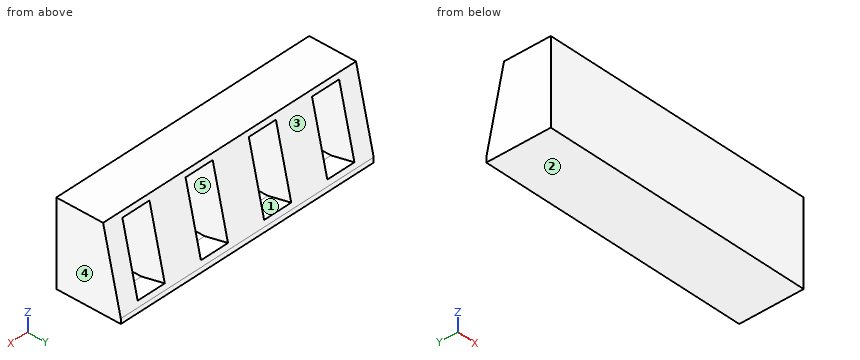
from build123d import *

# Parameters (mm, degrees)
SKETCH1_W           = 711.2
SKETCH1_H           = 167.132
BOSS_EXTRUDE2_DEPTH = 203.2
CUT_EXTRUDE3_DEPTH  = 919.48
SKETCH6_W           = 76.2
SKETCH6_H           = 180.34
CUT_EXTRUDE5_DEPTH  = 114.3
SKETCH7_W           = 711.2
SKETCH7_H           = 167.132
BOSS_EXTRUDE3_DEPTH = 12.7


with BuildPart() as part:
    # Sketch1 → Boss-Extrude2 (new body)
    with BuildSketch(Plane.XY):
        with Locations((355.6, 83.566)):
            Rectangle(SKETCH1_W, SKETCH1_H)
    extrude(amount=BOSS_EXTRUDE2_DEPTH)

    # Sketch5 → Cut-Extrude3 (cut)
    with BuildSketch(Plane(origin=(711.2, 0, 0), x_dir=(0, 0, -1), z_dir=(1, 0, 0))):
        Polygon((0, 167.132), (-203.2, 121.275720121), (-203.2, 167.132), align=None)
    extrude(amount=-CUT_EXTRUDE3_DEPTH, mode=Mode.SUBTRACT)

    # Sketch6 → Cut-Extrude5 (cut)
    with BuildSketch(Plane(origin=(0, 159.032892036, 35.88905909), x_dir=(1, 0, 0), z_dir=(0, 0.9754694514544971, 0.22013484340072725))):
        with Locations((266.7, -67.363402116)):
            Rectangle(SKETCH6_W, SKETCH6_H)
        with Locations((88.9, -67.363402116)):
            Rectangle(SKETCH6_W, SKETCH6_H)
        with Locations((444.5, -67.363402116)):
            Rectangle(SKETCH6_W, SKETCH6_H)
        with Locations((622.3, -67.363402116)):
            Rectangle(SKETCH6_W, SKETCH6_H)
    extrude(amount=-CUT_EXTRUDE5_DEPTH, mode=Mode.SUBTRACT)

    # Sketch7 → Boss-Extrude3 (add)
    with BuildSketch(Plane(origin=(0, 0, 0), x_dir=(-1, 0, 0), z_dir=(0, 0, -1))):
        with Locations((-355.6, 83.566)):
            Rectangle(SKETCH7_W, SKETCH7_H)
    extrude(amount=BOSS_EXTRUDE3_DEPTH)


solid = part.part
Could you check a few things on this model? Use its own coordinates, in mm. Face numbers are marked on the shaded views. A direction names the side the tool comes from. Coordinates: 2 decimals unless noted, no trailing zeros. Order: outer loops, then holes, each group sorted by start corner. A loop starts at its lowest first (then second) coordinate and runs counter-clockwise, first axis right, second up. Notation, with made-up numbers: (68.25, 85.25) - (92.25, 85.25) arc R13 ccw to (92.25, 100.25) - close; hole circle Ø11 at (11, -1.75). An arc over 180 degrees is marked (long way). Answer in a Markdown table with one row per item. Add a question column.
(1) I need wall thicknesses on L1, parallel to X at y = 81.5, z = 98.5; L2, parallel to Z at x = 298, y = 105; L3, parallel to Z at x = 103, y = 86. Which ranges of each line are inside material? Lowest first, please.
(2) If we section it at C-C, the plane z = 57.5: Please give me the cut outline in (x, y).
(3) If we section it at A-A, the plane x = 253: Please give me the cut outline in (y, z).
(4) If we section it at D-D, the plane y = 144: Please give me the cut outline in (x, z), then the cut area to 3 significant figures.
(5) If we mould it in two halves opening along X, with no side actions, what happens to the marked faces 3, 4 and 5? For each: released by +X, released by -X, zero draft, split by the parting line, or undercut.
(6) On a 3-axis mill with a long thin cutter (end or side, diameter ignored), from which of +Z, -Z, +X, -X, +Y, -Y can I reach the whole of each face in a straight line? I mean the marked faces 1 and 2. Say none if no direction works.
(7) If we section it at B-B, the plane y = 79.5: Please give me the cut outline in (x, z).
(8) Will these pins go through, and if not, where does the flat tip stop? pin 1 (10 mm diameter, centred on x = 301, z = 172, fed in from +Y); pin 2 (4 mm diameter, centred on x = 550.5, z = 10, fed in from +Y); pin 3 (12 mm diameter, centred on y = 141, z = 145.5, fed in from -X); pin 4 (1.5 mm diameter, centred on x = 520, z = 103, fed in from +Y).
Results are:
| question | item | result |
|---|---|---|
| 1 | L1 | x = 0 to 50.8, 127 to 228.6, 304.8 to 406.4, 482.6 to 584.2, 660.4 to 711.2 |
| 1 | L2 | z = -12.7 to 0.32, 185.19 to 203.2 |
| 1 | L3 | z = -12.7 to 0, 180.9 to 203.2 |
| 2 | outline | (0, 0) - (711.2, 0) - (711.2, 154.16) - (660.4, 154.16) - (660.4, 36.98) - (584.2, 36.98) - (584.2, 154.16) - (482.6, 154.16) - (482.6, 36.98) - (406.4, 36.98) - (406.4, 154.16) - (304.8, 154.16) - (304.8, 36.98) - (228.6, 36.98) - (228.6, 154.16) - (127, 154.16) - (127, 36.98) - (50.8, 36.98) - (50.8, 154.16) - (0, 154.16) - close |
| 3 | outline | (0, -12.7) - (167.13, -12.7) - (167.13, 0) - (164.05, 13.64) - (103.6, 0) - (49.96, 0) - (12.86, 164.4) - (124.35, 189.56) - (121.28, 203.2) - (0, 203.2) - close |
| 4 | outline | (0, -12.7) - (711.2, -12.7) - (711.2, 102.5) - (660.4, 102.5) - (660.4, 9.12) - (584.2, 9.12) - (584.2, 102.5) - (482.6, 102.5) - (482.6, 9.12) - (406.4, 9.12) - (406.4, 102.5) - (304.8, 102.5) - (304.8, 9.12) - (228.6, 9.12) - (228.6, 102.5) - (127, 102.5) - (127, 9.12) - (50.8, 9.12) - (50.8, 102.5) - (0, 102.5) - close |
| 4 | area | 53,500 mm2 |
| 5 | face 3 | zero draft |
| 5 | face 4 | released by +X |
| 5 | face 5 | undercut |
| 6 | face 1 | none |
| 6 | face 2 | -Z, +X, -X, +Y, -Y |
| 7 | outline | (0, -12.7) - (711.2, -12.7) - (711.2, 203.2) - (0, 203.2) - close; hole (50.8, 0) - (127, 0) - (127, 179.44) - (50.8, 179.44) - close; hole (228.6, 0) - (304.8, 0) - (304.8, 179.44) - (228.6, 179.44) - close; hole (406.4, 0) - (482.6, 0) - (482.6, 179.44) - (406.4, 179.44) - close; hole (584.2, 0) - (660.4, 0) - (660.4, 179.44) - (584.2, 179.44) - close |
| 8 | pin 1 | stops at y = 129.05 |
| 8 | pin 2 | stops at y = 165.33 |
| 8 | pin 3 | passes through |
| 8 | pin 4 | stops at y = 144.06 |
